Can you work these out from the model? Positions are in its coordinate system, mm. A direction names the side the tool comes from. Give positions to 0.01 mm unless a question says otherwise; leave off trailing zeros. Loops run counter-clockwise (first coordinate to the right, second up) from the corner with the lowest first, then second, coordinate; pieces in that order, holes last. Notation, with made-up numbers: (14.25, 36.25) -> (46.25, 36.25) arc R17 cw to (46.25, 68.25) -> close; hole circle Ø8 at (-6, 16.25). An arc over 180 degrees is marked (long way). Return JSON: item names as keys, results as strings. Group by question number.
Q1. I need wall thicknesses on line 1 along X through (y, z) = (0.4, 4); line 2 along X through (y, z) = (1.95, 0); line 3 along Y through (x, z) = (-11, 0.25). Which ranges of each line are inside material? Lowest first, please. Write a range as [from, to].
Q2. Suppose I cut it at A-A, the plane x = -23. Please give me the cut outline in (y, z), and give its area (3 significant figures).
Q3. Which directions (+Z, -Z, +X, -X, +Y, -Y) give clear straight access to the entire face, cutting with the end or side of a thin tool? Please do faces 5 (the flat face through (15.9, 0.5, 8)), 6 (the flat face through (6.4, 0.5, 0)), 7 (the flat face through (4, 0.5, -10.5)).
Q4. Suppose I cut it at B-B, the plane z = 4. Please give me the cut outline in (x, y).
Q5. Thinking about a two-plate mould opening in X: for faces 1 (the cylindrical face through (9.76, 1.52, -2.17)), 2 (the flat face through (26, 0.5, 4.1)), 3 (the flat face through (-17.9, 0.5, 0)), 4 (the flat face through (-0.1, 0.5, 8)), which applies, pulls with the +X half, pulls with the -X half, needs draft (parallel to the pull), parting line crosses it, or undercut?
Q6. Suppose I cut it at C-C, the plane x = 0. Please give me the cut outline in (y, z).
Q7. Suppose I cut it at D-D, the plane z = -3.25. Please give me the cut outline in (x, y).
Q8. Will these pins go through, and if not, where does the flat tip stop? pin 1 (1.1 mm diameter, centred on y = 0.5, z = -10, fed in from -X); pin 2 (0.8 mm diameter, centred on x = -14.5, y = 0.5, fed in from +Z); pin 3 (12 mm diameter, centred on x = 2, z = -8, fed in from +Y).
```python
from build123d import *

# Parameters (mm, degrees)
SKETCH_2_R      = 1.9
EXTRUDE_1_DEPTH = 1


with BuildPart() as part:
    # Эскиз1 → Повернуть1 (revolve)
    with BuildSketch(Plane.XY, mode=Mode.PRIVATE) as revolve_1_sk:
        with BuildLine():
            Line((8.8, 0), (10, 0))
            Line((10, 0), (10, 3))
            ThreePointArc((10, 3), (7.071067812, 10.071067812), (0, 13))
            Line((0, 13), (0, 11.8))
            ThreePointArc((0, 11.8), (6.222539674, 9.222539674), (8.8, 3))
            Line((8.8, 3), (8.8, 0))
        make_face()
    revolve(revolve_1_sk.sketch.rotate(Axis((0, 13, 0), (0, -1, 0)), 90), axis=Axis((0, 13, 0), (0, -1, 0)))

    # Эскиз2 → Бобышка-Вытянуть1 (add)
    # profile 1 of 3: a face of its own
    with BuildSketch(Plane(origin=(0, 0, 0), x_dir=(1, 0, 0), z_dir=(0, 1, 0))):
        Polygon((0, -8), (0, 0), (-4, 0), (-26, 0), (-26, -8), align=None)
        with Locations(Location((-23, -4, 0), (0, 0, 270))):
            Circle(SKETCH_2_R, mode=Mode.SUBTRACT)
    # profile 2 of 3: a face of its own
    with BuildSketch(Plane(origin=(0, 0, 0), x_dir=(1, 0, 0), z_dir=(0, 1, 0))):
        Polygon((26, -8), (26, 0), (4, 0), (0, 0), (0, -8), align=None)
        with Locations(Location((23, -4, 0), (0, 0, 270))):
            Circle(SKETCH_2_R, mode=Mode.SUBTRACT)
    # profile 3 of 3: a face of its own
    with BuildSketch(Plane(origin=(0, 0, 0), x_dir=(1, 0, 0), z_dir=(0, 1, 0))):
        Polygon((0, 0), (4, 0), (4, 11.9), (-4, 11.9), (-4, 0), align=None)
    extrude(amount=EXTRUDE_1_DEPTH)


solid = part.part
```
Ans:
{
 "1": {"line 1": "x = [-26, -24.9], [-21.1, 21.1], [24.9, 26]", "line 2": "x = [-10, -8.8], [8.8, 10]", "line 3": "y = [0, 1]"},
 "2": {"outline": "(0, 0) -> (1, 0) -> (1, 2.1) -> (0, 2.1) -> close; (0, 5.9) -> (1, 5.9) -> (1, 8) -> (0, 8) -> close", "area": "4.20 mm^2"},
 "3": {"face 5": "+Z, +X, +Y, -Y", "face 6": "-Y", "face 7": "-Z, +X, +Y, -Y"},
 "4": {"outline": "(-26, 0) -> (-24.9, 0) -> (-24.9, 1) -> (-26, 1) -> close; (-21.1, 0) -> (21.1, 0) -> (21.1, 1) -> (9.17, 1) -> (9.17, 3) arc R9.17 ccw to (-9.17, 3) -> (-9.17, 1) -> (-21.1, 1) -> close; (24.9, 0) -> (26, 0) -> (26, 1) -> (24.9, 1) -> close; hole (-7.84, 1) -> (7.84, 1) -> (7.84, 3) arc R7.84 ccw to (-7.84, 3) -> close"},
 "5": {"face 1": "parting line crosses it", "face 2": "pulls with the +X half", "face 3": "needs draft", "face 4": "undercut"},
 "6": {"outline": "(0, -11.9) -> (1, -11.9) -> (1, -10) -> (3, -10) arc R10 ccw to (3, 10) -> (0, 10) -> (0, 8.8) -> (3, 8.8) arc R8.8 cw to (3, -8.8) -> (1, -8.8) -> (1, 8) -> (0, 8) -> close"},
 "7": {"outline": "(-9.46, 0) -> (-8.18, 0) -> (-8.18, 3) arc R8.18 cw to (8.18, 3) -> (8.18, 0) -> (9.46, 0) -> (9.46, 3) arc R9.46 ccw to (-9.46, 3) -> close; (-4, 0) -> (4, 0) -> (4, 1) -> (-4, 1) -> close"},
 "8": {"pin 1": "stops at x = -4", "pin 2": "stops at z = 8", "pin 3": "stops at y = 12.74"}
}
